```python
from build123d import *

# Parameters (mm, degrees)
MODEL_W         = 63.70079
MODEL_H         = 43.04936
MODEL_R         = 1.6
EXTRUDE_1_DEPTH = 3


with BuildPart() as part:
    # Model → 凸台-拉伸1 (new body)
    with BuildSketch(Plane.XY):
        with Locations((31.869154462, 21.443783961)):
            Rectangle(MODEL_W, MODEL_H)
        with Locations((22.344199462, 21.443163961)):
            Circle(MODEL_R, mode=Mode.SUBTRACT)
        with Locations((41.394099462, 21.443163961)):
            Circle(MODEL_R, mode=Mode.SUBTRACT)
        Polygon((43.919449462, 18.918563961), (43.919449462, 17.918163961), (43.118649462, 17.918163961), (43.118649462, 14.818963961), (43.919449462, 14.818963961), (43.919449462, 9.018753961), (43.118649462, 9.018753961), (43.118649462, 5.918193961), (43.919449462, 5.918193961), (43.919449462, 4.919103961), (57.918749462, 4.919103961), (57.918749462, 5.918193961), (58.719549462, 5.918193961), (58.719549462, 9.018753961), (57.918749462, 9.018753961), (57.918749462, 14.818963961), (58.719549462, 14.818963961), (58.719549462, 17.918163961), (57.918749462, 17.918163961), (57.918749462, 18.918563961), align=None, mode=Mode.SUBTRACT)
        Polygon((24.869449462, 18.918563961), (24.869449462, 17.918163961), (24.068749462, 17.918163961), (24.068749462, 14.818963961), (24.869449462, 14.818963961), (24.869449462, 9.018753961), (24.068749462, 9.018753961), (24.068749462, 5.918193961), (24.869449462, 5.918193961), (24.869449462, 4.919103961), (38.868749462, 4.919103961), (38.868749462, 5.918193961), (39.669549462, 5.918193961), (39.669549462, 9.018753961), (38.868749462, 9.018753961), (38.868749462, 14.818963961), (39.669549462, 14.818963961), (39.669549462, 17.918163961), (38.868749462, 17.918163961), (38.868749462, 18.918563961), align=None, mode=Mode.SUBTRACT)
        Polygon((5.819399462, 18.918563961), (5.819399462, 17.918163961), (5.018759462, 17.918163961), (5.018759462, 14.818963961), (5.819399462, 14.818963961), (5.819399462, 9.018753961), (5.018759462, 9.018753961), (5.018759462, 5.918193961), (5.819399462, 5.918193961), (5.819399462, 4.919103961), (19.818949462, 4.919103961), (19.818949462, 5.918193961), (20.619549462, 5.918193961), (20.619549462, 9.018753961), (19.818949462, 9.018753961), (19.818949462, 14.818963961), (20.619549462, 14.818963961), (20.619549462, 17.918163961), (19.818949462, 17.918163961), (19.818949462, 18.918563961), align=None, mode=Mode.SUBTRACT)
        Polygon((43.919449462, 37.968463961), (43.919449462, 36.968163961), (43.118649462, 36.968163961), (43.118649462, 33.868963961), (43.919449462, 33.868963961), (43.919449462, 28.068763961), (43.118649462, 28.068763961), (43.118649462, 24.968163961), (43.919449462, 24.968163961), (43.919449462, 23.969063961), (57.918749462, 23.969063961), (57.918749462, 24.968163961), (58.719549462, 24.968163961), (58.719549462, 28.068763961), (57.918749462, 28.068763961), (57.918749462, 33.868963961), (58.719549462, 33.868963961), (58.719549462, 36.968163961), (57.918749462, 36.968163961), (57.918749462, 37.968463961), align=None, mode=Mode.SUBTRACT)
        Polygon((24.869449462, 37.968463961), (24.869449462, 36.968163961), (24.068749462, 36.968163961), (24.068749462, 33.868963961), (24.869449462, 33.868963961), (24.869449462, 28.068763961), (24.068749462, 28.068763961), (24.068749462, 24.968163961), (24.869449462, 24.968163961), (24.869449462, 23.969063961), (38.868749462, 23.969063961), (38.868749462, 24.968163961), (39.669549462, 24.968163961), (39.669549462, 28.068763961), (38.868749462, 28.068763961), (38.868749462, 33.868963961), (39.669549462, 33.868963961), (39.669549462, 36.968163961), (38.868749462, 36.968163961), (38.868749462, 37.968463961), align=None, mode=Mode.SUBTRACT)
        Polygon((5.819399462, 37.968463961), (5.819399462, 36.968163961), (5.018759462, 36.968163961), (5.018759462, 33.868963961), (5.819399462, 33.868963961), (5.819399462, 28.068763961), (5.018759462, 28.068763961), (5.018759462, 24.968163961), (5.819399462, 24.968163961), (5.819399462, 23.969063961), (19.818949462, 23.969063961), (19.818949462, 24.968163961), (20.619549462, 24.968163961), (20.619549462, 28.068763961), (19.818949462, 28.068763961), (19.818949462, 33.868963961), (20.619549462, 33.868963961), (20.619549462, 36.968163961), (19.818949462, 36.968163961), (19.818949462, 37.968463961), align=None, mode=Mode.SUBTRACT)
    extrude(amount=EXTRUDE_1_DEPTH)


solid = part.part
```
Geometry check sheet. Reference: the model listing, model coordinates, mm. A direction names the side the tool comes from. Coordinates: 2 decimals unless noted, no trailing zeros. Loops run counter-clockwise (first coordinate to the right, second up) from the corner with the lowest first, then second, coordinate; pieces in that order, holes last. Notation, with made-up numbers: (1.25, 82) - (55.25, 82) arc R33 cw to (55.25, 111) - close; hole circle Ø2 at (-9, 79.25). An arc over 180 degrees is marked (long way). One line per item, written item: value. Start each with the question number.
(1) Tool access check on faces 4 (the flat face through (63.72, 21, 1)), 5 (the flat face through (43.919, 31, 1)). Record the directions out of +Z, -Z, +X, -X, +Y, -Y that give a thin tool (end or side, any length) a straight path to the whole face; none if there is none.
(2) Cross-section at B-B on z = 0.9. Count the separate pieces of the cut face and the enclosed holes in it, plus the area to 3 significant figures.
(3) Mould release check, pull along Y, two halves, no side actions. Record for faces 1 (the flat face through (31, -0.081, 1)), 2 (the flat face through (24.069, 7, 1)), 3 (the flat face through (31, 22, 0)): released by +Y, released by -Y, zero draft, split by the parting line, or undercut.
(4) Material ranges on line 1 (Y direction, x = 53.5, z = 0.8); line 2 (Y direction, x = 39, z = 2.2); line 3 (X direction, y = 16, z = 2.4), recorded low to high. Write a range as [from, to].
(5) Depth check by flat-ended pin: P1, Ø5, axis at x = 16, y = 8.5, coming from the +Z side. Enter the tip coordinate at first touch or a pass-through.
(6) Cross-section at A-A on x = 33. Enter the section's corners in (y, z), plus the area to 3 significant figures.
Results below:
1. face 4: +Z, -Z, +X, +Y, -Y
1. face 5: +Z, -Z
2. separate pieces: 1
2. enclosed holes: 8
2. area: 1,490 mm2
3. face 1: released by -Y
3. face 2: undercut
3. face 3: zero draft
4. line 1: y = [-0.08, 4.92], [18.92, 23.97], [37.97, 42.97]
4. line 2: y = [-0.08, 5.92], [9.02, 14.82], [17.92, 24.97], [28.07, 33.87], [36.97, 42.97]
4. line 3: x = [0.02, 5.02], [20.62, 24.07], [39.67, 43.12], [58.72, 63.72]
5. P1: passes through
6. outline: (-0.08, 0) - (4.92, 0) - (4.92, 3) - (-0.08, 3) - close; (18.92, 0) - (23.97, 0) - (23.97, 3) - (18.92, 3) - close; (37.97, 0) - (42.97, 0) - (42.97, 3) - (37.97, 3) - close
6. area: 45.2 mm2
